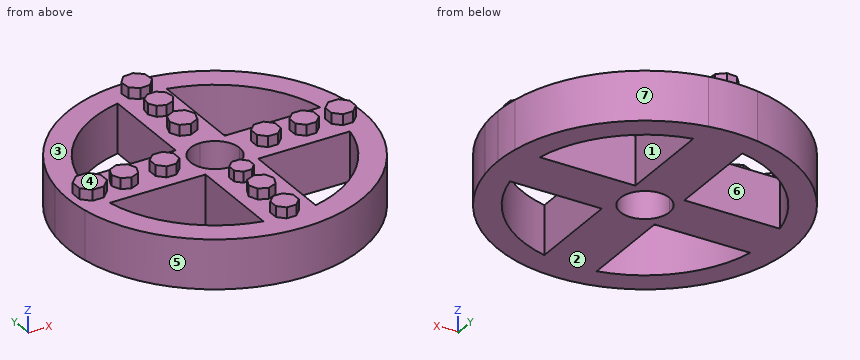
from build123d import *

# Parameters (mm, degrees)
F1_DEPTH = 12.7
F3_DEPTH = 5.588


with BuildPart() as f1:
    # F0 (on Top) → F1 (new body, symmetric)
    with BuildSketch(Plane.XY):
        with BuildLine():
            ThreePointArc((75.134213, -12.7), (75.933086, -6.372321), (76.2, 0))
            ThreePointArc((76.2, 0), (75.933086, 6.372321), (75.134213, 12.7))
            ThreePointArc((75.134213, 12.7), (53.881537, 53.881537), (12.7, 75.134213))
            ThreePointArc((12.7, 75.134213), (0, 76.2), (-12.7, 75.134213))
            ThreePointArc((-12.7, 75.134213), (-53.881537, 53.881537), (-75.134213, 12.7))
            ThreePointArc((-75.134213, 12.7), (-76.2, 0), (-75.134213, -12.7))
            ThreePointArc((-75.134213, -12.7), (0, -76.2), (75.134213, -12.7))
        make_face()
        with BuildLine():
            ThreePointArc((-12.690558, -62.218966), (-44.897873, -44.904687), (-62.217039, -12.7))
            Line((-62.217039, -12.7), (-12.690558, -12.817428))
            Line((-12.690558, -12.817428), (-12.690558, -62.218966))
        make_face(mode=Mode.SUBTRACT)
        with BuildLine():
            Line((14.67346, -12.7), (62.217039, -12.7))
            ThreePointArc((62.217039, -12.7), (45.610118, -44.181073), (14.67346, -61.781385))
            Line((14.67346, -61.781385), (14.67346, -12.7))
        make_face(mode=Mode.SUBTRACT)
        with BuildLine():
            Line((-12.7, 12.7), (-62.217039, 12.7))
            ThreePointArc((-62.217039, 12.7), (-44.901281, 44.901281), (-12.7, 62.217039))
            Line((-12.7, 62.217039), (-12.7, 12.7))
        make_face(mode=Mode.SUBTRACT)
        with BuildLine():
            ThreePointArc((0, 12.7), (8.980256, 8.980256), (12.7, 0))
            ThreePointArc((12.7, 0), (0, -12.7), (-12.7, 0))
            ThreePointArc((-12.7, 0), (-8.980256, 8.980256), (0, 12.7))
        make_face(mode=Mode.SUBTRACT)
        with BuildLine():
            Line((12.7, 12.7), (12.7, 62.217039))
            ThreePointArc((12.7, 62.217039), (44.901281, 44.901281), (62.217039, 12.7))
            Line((62.217039, 12.7), (12.7, 12.7))
        make_face(mode=Mode.SUBTRACT)
    extrude(amount=F1_DEPTH, both=True)

    # F2 (on face) → F3 (join)
    with BuildSketch(Plane.XY.offset(12.7)):
        Polygon((3.232429, 60.705414), (6.682069, 64.812133), (6.217445, 70.155287), (2.110725, 73.604928), (-3.232429, 73.140303), (-6.682069, 69.033583), (-6.217445, 63.69043), (-2.110725, 60.240789), align=None)
        Polygon((2.237321, 54.034017), (-2.237321, 54.034017), (-5.665096, 51.157772), (-6.44211, 46.751109), (-4.204789, 42.875955), (0, 41.345537), (4.204789, 42.875955), (6.44211, 46.751109), (5.665096, 51.157772), align=None)
        Polygon((4.574757, 33.132439), (-0.353307, 34.881021), (-5.074409, 32.632787), (-6.822991, 27.704723), (-4.574757, 22.983621), (0.353307, 21.235039), (5.074409, 23.483272), (6.822991, 28.411337), align=None)
        Polygon((-57.702381, -2.95684), (-57.702381, 2.95684), (-61.883984, 7.138442), (-67.797663, 7.138442), (-71.979266, 2.95684), (-71.979266, -2.95684), (-67.797663, -7.138442), (-61.883984, -7.138442), align=None)
        Polygon((-51.800584, 4.580097), (-53.689675, -0.019427), (-51.77311, -4.607571), (-47.173586, -6.496662), (-42.585442, -4.580097), (-40.696351, 0.019427), (-42.612916, 4.607571), (-47.21244, 6.496662), align=None)
        Polygon((-32.313216, 2.565593), (-32.32931, -2.526738), (-28.739868, -6.138941), (-23.647537, -6.155035), (-20.035334, -2.565593), (-20.01924, 2.526738), (-23.608682, 6.138941), (-28.701014, 6.155035), align=None)
        Polygon((-5.155539, -20.568707), (-5.155539, -24.839695), (-2.135494, -27.85974), (2.135494, -27.85974), (5.155539, -24.839695), (5.155539, -20.568707), (2.135494, -17.548662), (-2.135494, -17.548662), align=None)
        Polygon((-4.566506, -34.879606), (-6.537733, -39.479133), (-4.679244, -44.125357), (-0.079718, -46.096583), (4.566506, -44.238094), (6.537733, -39.638568), (4.679244, -34.992344), (0.079718, -33.021117), align=None)
        Polygon((-5.948699, -56.923812), (-5.948699, -61.851876), (-2.464032, -65.336543), (2.464032, -65.336543), (5.948699, -61.851876), (5.948699, -56.923812), (2.464032, -53.439145), (-2.464032, -53.439145), align=None)
        Polygon((20.225577, 2.546165), (20.225577, -2.546165), (23.826398, -6.146986), (28.918728, -6.146986), (32.519549, -2.546165), (32.519549, 2.546165), (28.918728, 6.146986), (23.826398, 6.146986), align=None)
        Polygon((40.054575, 2.546165), (40.054575, -2.546165), (43.655396, -6.146986), (48.747726, -6.146986), (52.348547, -2.546165), (52.348547, 2.546165), (48.747726, 6.146986), (43.655396, 6.146986), align=None)
        Polygon((58.693826, 2.628301), (58.693826, -2.628301), (62.410805, -6.34528), (67.667407, -6.34528), (71.384385, -2.628301), (71.384385, 2.628301), (67.667407, 6.34528), (62.410805, 6.34528), align=None)
    extrude(amount=F3_DEPTH)


solid = f1.part
Here's how the part is built. I have some questions about the finished solid (model axes, mm). Face numbers are marked on the shaded views. A direction names the side the tool comes from. Round coordinates to 2 decimals unless told otherwise and drop trailing zeros. Write each loop counter-clockwise with the first axis right and the second up, starting at its lowest first coordinate (ties: lowest second). Pieces come first, ordered by that corner, then holes.
1. For the marked faces 1, 2 and 3, which set-ups out of +Z, -Z, +X, -X, +Y, -Y let a thin tool reach every point of the face, with its end or its side?
2. I need wall thicknesses on L1, parallel to Y at x = 42, z = 12.5; L2, parallel to X at y = -55.5, z = 5; L3, parallel to X at y = 50.5, z = 7.5. Which ranges of each line are inside material? Lowest first, please.
3. If we mould it in two halves opening along X, with no side actions, what happens to the marked faces 4, 5, 6 and 7? For each: released by +X, released by -X, zero draft, split by the parting line, or undercut.
4. Suppose I cut it at B-B (y = 49). List the corners of the cut face in (x, z) for me, and give its area (3 significant figures).
5. Suppose I cut it at C-C (x = 56.5). List the corners of the cut face in (y, z) for me.
6. Suppose I cut it at D-D (x = 26). List the corners of the cut face in (y, z) for me.
7. Will these pins go through, and if not, where does the flat tip stop? pin 1 Ø5 at (y, z) = (-50, -2) entering from -X; pin 2 Ø2.5 at (x, z) = (45, 17) entering from -Y; pin 3 Ø4.5 at (x, z) = (-63.5, 16.5) entering from +Y.
8. Suppose I cut it at A-A (z = 8). List the corners of the cut face in (x, y) for me.
Answer sheet:
1. face 1: +Z, -Z
1. face 2: -Z, +X, -X, +Y, -Y
1. face 3: +Z
2. L1: y = -63.58 to -47.63, -12.7 to 12.7, 47.63 to 63.58
2. L2: x = -52.21 to -30.85, -12.69 to 14.67, 30.85 to 52.21
2. L3: x = -57.06 to -38.5, -12.7 to 12.7, 38.5 to 57.06
3. face 4: zero draft
3. face 5: split by the parting line
3. face 6: undercut
3. face 7: released by +X
4. outline: (-58.36, -12.7) - (-40.39, -12.7) - (-40.39, 12.7) - (-58.36, 12.7) - close; (-12.7, -12.7) - (12.7, -12.7) - (12.7, 12.7) - (6.05, 12.7) - (6.05, 18.29) - (-6.05, 18.29) - (-6.05, 12.7) - (-12.7, 12.7) - close; (40.39, -12.7) - (58.36, -12.7) - (58.36, 12.7) - (40.39, 12.7) - close
4. area: 1,630 mm2
5. outline: (-51.13, -12.7) - (-28.98, -12.7) - (-28.98, 12.7) - (-51.13, 12.7) - close; (-12.7, -12.7) - (12.7, -12.7) - (12.7, 12.7) - (-12.7, 12.7) - close; (28.98, -12.7) - (51.13, -12.7) - (51.13, 12.7) - (28.98, 12.7) - close
6. outline: (-71.63, -12.7) - (-57.93, -12.7) - (-57.93, 12.7) - (-71.63, 12.7) - close; (-12.7, -12.7) - (12.7, -12.7) - (12.7, 12.7) - (6.15, 12.7) - (6.15, 18.29) - (-6.15, 18.29) - (-6.15, 12.7) - (-12.7, 12.7) - close; (57.93, -12.7) - (71.63, -12.7) - (71.63, 12.7) - (57.93, 12.7) - close
7. pin 1: stops at x = -59.58
7. pin 2: stops at y = -6.15
7. pin 3: stops at y = 7.14
8. outline: (-75.13, -12.7) arc R76.2 ccw to (75.13, -12.7) arc R76.2 ccw to (76.2, 0) arc R76.2 ccw to (75.13, 12.7) arc R76.2 ccw to (12.7, 75.13) arc R76.2 ccw to (-12.7, 75.13) arc R76.2 ccw to (-75.13, 12.7) arc R76.2 ccw to start; hole (-62.22, -12.7) arc R63.5 ccw to (-12.69, -62.22) - (-12.69, -12.82) - close; hole (-62.22, 12.7) - (-12.7, 12.7) - (-12.7, 62.22) arc R63.5 ccw to start; hole circle Ø25.4 at (0, 0); hole (12.7, 12.7) - (62.22, 12.7) arc R63.5 ccw to (12.7, 62.22) - close; hole (14.67, -61.78) arc R63.5 ccw to (62.22, -12.7) - (14.67, -12.7) - close
